```python
from build123d import *

# Parameters (mm, degrees)
BOSS_EXTRUDE1_DEPTH = 30
SKETCH2_R           = 5
CUT_EXTRUDE2_DEPTH  = 40
SKETCH4_R           = 5
CUT_EXTRUDE3_DEPTH  = 40


with BuildPart() as part:
    # Sketch1 → Boss-Extrude1 (new body)
    with BuildSketch(Plane.XY):
        Polygon((0, 0), (30, 0), (30, -60), (80, -60), (80, -80), (30, -80), (0, -80), align=None)
    extrude(amount=BOSS_EXTRUDE1_DEPTH)

    # Sketch2 → Cut-Extrude2 (cut)
    with BuildSketch(Plane(origin=(30, 0, 0), x_dir=(0, 0, -1), z_dir=(1, 0, 0))):
        with Locations((-15, -25)):
            Circle(SKETCH2_R)
    extrude(amount=-CUT_EXTRUDE2_DEPTH, mode=Mode.SUBTRACT)

    # Sketch4 → Cut-Extrude3 (cut)
    with BuildSketch(Plane(origin=(0, -60, 0), x_dir=(1, 0, 0), z_dir=(0, 1, 0))):
        with Locations(Location((50, -15, 0), (0, 0, 270))):
            Circle(SKETCH4_R)
    extrude(amount=-CUT_EXTRUDE3_DEPTH, mode=Mode.SUBTRACT)


solid = part.part
```
Verification items for the finished model (mm, model axes). A direction names the side the tool comes from. Coordinates: 2 decimals unless noted, no trailing zeros. Loops run counter-clockwise (first coordinate to the right, second up) from the corner with the lowest first, then second, coordinate; pieces in that order, holes last. Notation, with made-up numbers: (-37, 77.25) - (10, 77.25) arc R24 ccw to (10, 110.25) - close; hole circle Ø6 at (-23.75, -23). An arc over 180 degrees is marked (long way). Return JSON: item names as keys, results as strings.
1. Section check A-A, the plane z = 15. Record the boundary of the cut face in (x, y), then the cut area to 3 significant figures.
Established:
{"outline": "(0, -80) - (45, -80) - (45, -60) - (30, -60) - (30, -30) - (0, -30) - close; (0, -20) - (30, -20) - (30, 0) - (0, 0) - close; (55, -80) - (80, -80) - (80, -60) - (55, -60) - close", "area": "2,900 mm2"}
2. Go/stop test with a flat-tipped pin: pin 1 (8 mm diameter, centred on x = 37.5, z = 26, fed in from +Y). Record where the tip stops, or that it passes through.
Established:
{"pin 1": "stops at y = -60"}
3. Section check B-B, the plane x = 50. Record the boundary of the cut face in (y, z).
Established:
{"outline": "(-80, 0) - (-60, 0) - (-60, 10) - (-80, 10) - close; (-80, 20) - (-60, 20) - (-60, 30) - (-80, 30) - close"}
4. Section check C-C, the plane x = 20. Record the boundary of the cut face in (y, z).
Established:
{"outline": "(-80, 0) - (0, 0) - (0, 30) - (-80, 30) - close; hole circle Ø10 at (-25, 15)"}
5. Section check D-D, the plane y = -67. Record the boundary of the cut face in (x, z), then the cut area to 3 significant figures.
Established:
{"outline": "(0, 0) - (80, 0) - (80, 30) - (0, 30) - close; hole circle Ø10 at (50, 15)", "area": "2,320 mm2"}
6. Thickness scan on L1, parallel to X at y = -73, z = 15; L2, parallel to Y at x = 9.75, z = 15; L3, parallel to X at y = -56, z = 11.25. Record the ranges inside material, lowest first.
Established:
{"L1": "x = 0 to 45, 55 to 80", "L2": "y = -80 to -30, -20 to 0", "L3": "x = 0 to 30"}
7. Tool access check on faces 1 (the flat face through (30, -30, 18)), 2 (the flat face through (15, 0, 15)). Record the directions out of +Z, -Z, +X, -X, +Y, -Y that give a thin tool (end or side, any length) a straight path to the whole face; none if there is none.
Established:
{"face 1": "+Z, -Z, +X, +Y", "face 2": "+Z, -Z, +X, -X, +Y"}
8. Mould release check, pull along Z, two halves, no side actions. Record for faces 3 (the flat face through (23, -48, 30)), 4 (the flat face through (80, -70, 15)), 5 (the cylindrical face through (15.21, -29.88, 16.08)): +Z half, -Z half, draft (parallel to the pull), parting line (faces both ways), or undercut.
Established:
{"face 3": "+Z half", "face 4": "draft", "face 5": "undercut"}
